Check sheet for the modelled part. Datum: model origin and axes. Units: mm. A direction names the side the tool comes from. Give positions to 0.01 mm unless a question says otherwise; leave off trailing zeros. Order: outer loops, then holes, each group sorted by start corner. A loop starts at its lowest first (then second) coordinate and runs counter-clockwise, first axis right, second up.
from build123d import *

# Parameters (mm, degrees)
SKETCH1_W               = 11.811
SKETCH1_H               = 3.175
SKETCH1_R               = 3.1623
BOSS_EXTRUDE1_DEPTH     = 5.08
BOSS_EXTRUDE2_OUTLINE_W = 16.150142566
BOSS_EXTRUDE2_OUTLINE_H = 6.574737844
BOSS_EXTRUDE2_DEPTH     = 12.7
BOSS_EXTRUDE3_START     = -5.08
BOSS_EXTRUDE3_DEPTH     = 5.08
BOSS_EXTRUDE5_DEPTH     = 2.032
BOSS_EXTRUDE6_START     = -1.27
SKETCH1_6_R             = 5.53085
SKETCH1_6_R_2           = 3.1623
BOSS_EXTRUDE6_DEPTH     = 1.27


# Read off the part's stored shape, not the designer's step: Boss-Extrude2
with BuildPart() as part:
    # Sketch1 → Boss-Extrude1 (new body)
    with BuildSketch(Plane(origin=(0, 0, 0), x_dir=(1, 0, 0), z_dir=(0, 1, 0))):
        with BuildLine():
            ThreePointArc((13.753578899, 4.597841674), (0, 5.078127233), (-13.753578899, 4.597841674))
            Line((-13.753578899, 4.597841674), (-13.39934665, -0.467915496))
            Line((-13.39934665, -0.467915496), (-13.39934665, -22.557024998))
            Line((-13.39934665, -22.557024998), (13.39934665, -22.557024998))
            Line((13.39934665, -22.557024998), (13.39934665, -0.467915496))
            Line((13.39934665, -0.467915496), (13.753578899, 4.597841674))
        make_face()
        with Locations((0, -3.5433)):
            Rectangle(SKETCH1_W, SKETCH1_H, mode=Mode.SUBTRACT)
        with Locations(Location((0, -13.62075, 0), (0, 0, 270))):
            Circle(SKETCH1_R, mode=Mode.SUBTRACT)
    extrude(amount=BOSS_EXTRUDE1_DEPTH)

    # Boss-Extrude2 outline → Boss-Extrude2 (add)
    with BuildSketch(Plane(origin=(0, 0, 0), x_dir=(1, 0, 0), z_dir=(0, 1, 0))):
        with Locations((0, -3.6068)):
            Rectangle(BOSS_EXTRUDE2_OUTLINE_W, BOSS_EXTRUDE2_OUTLINE_H)
        Polygon((-2.8321, -3.6068), (-2.8321, -5.1308), (-5.9055, -5.1308), (-5.9055, -1.9558), (5.9055, -1.9558), (5.9055, -5.1308), (2.8321, -5.1308), (2.8321, -3.6068), align=None, mode=Mode.SUBTRACT)
    extrude(amount=BOSS_EXTRUDE2_DEPTH)

    # Sketch1_4 → Boss-Extrude3 (add)
    with BuildSketch(Plane(origin=(0, 0, 0), x_dir=(1, 0, 0), z_dir=(0, 1, 0)).offset(BOSS_EXTRUDE3_START)):
        with BuildLine():
            ThreePointArc((-13.753578899, 4.597841674), (0, 5.078127233), (13.753578899, 4.597841674))
            Line((13.753578899, 4.597841674), (13.39934665, -0.467915496))
            ThreePointArc((13.39934665, -0.467915496), (6.703757073, -0.117014515), (0, 0))
            ThreePointArc((0, 0), (-6.703757073, -0.117014515), (-13.39934665, -0.467915496))
            Line((-13.39934665, -0.467915496), (-13.753578899, 4.597841674))
        make_face()
    extrude(amount=BOSS_EXTRUDE3_DEPTH)

    # Sketch2 → Boss-Extrude5 (add)
    with BuildSketch(Plane.XZ.offset(5.08)):
        Polygon((-13.753578899, -4.597841674), (-13.39934665, 0.467915496), (-13.300671129, 1.879041191), (13.300671129, 1.879041191), (13.39934665, 0.467915496), (13.753578899, -4.597841674), align=None)
    extrude(amount=-BOSS_EXTRUDE5_DEPTH)

    # Sketch1_6 → Boss-Extrude6 (add)
    with BuildSketch(Plane(origin=(0, 0, 0), x_dir=(1, 0, 0), z_dir=(0, 1, 0)).offset(BOSS_EXTRUDE6_START)):
        with Locations(Location((0, -13.62075, 0), (0, 0, 270))):
            Circle(SKETCH1_6_R)
        with Locations(Location((0, -13.62075, 0), (0, 0, 270))):
            Circle(SKETCH1_6_R_2, mode=Mode.SUBTRACT)
    extrude(amount=BOSS_EXTRUDE6_DEPTH)


solid = part.part
1) Material ranges on L1, parallel to X at y = 3, z = 3.75; L2, parallel to Y at x = 10, z = 1.75; L3, parallel to X at y = 2.5, z = 3.5, recorded low to high.
Recorded:
L1: x = -13.4 to -5.91, -2.83 to 2.83, 5.91 to 13.4
L2: y = -5.08 to -3.05, 0 to 5.08
L3: x = -13.4 to -5.91, 5.91 to 13.4
2) Section check C-C, the plane x = -4.5. Record the cut outline in (y, z).
Recorded:
outline: (-5.08, -5.03) - (5.08, -5.03) - (5.08, 0.32) - (12.7, 0.32) - (12.7, 1.96) - (0, 1.96) - (0, 0.05) - (-3.05, 0.05) - (-3.05, 1.88) - (-5.08, 1.88) - close; (-1.27, 10.41) - (0, 10.41) - (0, 5.13) - (12.7, 5.13) - (12.7, 6.89) - (5.08, 6.89) - (5.08, 22.56) - (0, 22.56) - (0, 16.84) - (-1.27, 16.84) - close
3) Set-up check for faces 1 (the face through (-13.399, 3, 11)), 2 (the face through (8.075, 9, 4)), 3 (the face through (-2.4, -1.27, 16)), 4 (the face through (-5.906, 6, 4)): record each of +Z, -Z, +X, -X, +Y, -Y from which the full face is reachable in a straight line by a thin tool's end or side.
Recorded:
face 1: +Z, -X, +Y, -Y
face 2: +Z, -Z, +X, +Y
face 3: +Z, +X, -X, -Y
face 4: +Y, -Y
4) Draft check along Z on faces 5 (the face through (0, 6, 3.607)), 6 (the face through (-0.19, -0.07, -5.08)), 7 (the face through (-8.075, 9, 4)). Enter one of: +Z half, -Z half, draft (parallel to the pull), parting line (faces both ways), or undercut.
Recorded:
face 5: undercut
face 6: -Z half
face 7: draft
5) Depth check by flat-ended pin: pin 1 Ø1.2 at (y, z) = (5.5, 4.5) entering from -X; pin 2 Ø5 at (x, z) = (1.5, 15.5) entering from +Y; pin 3 Ø4 at (y, z) = (0.5, 15) entering from +X. Enter the tip coordinate at first touch or a pass-through.
Recorded:
pin 1: stops at x = -13.4
pin 2: stops at y = 5.08
pin 3: stops at x = 13.4
6) Section check B-B, the plane y = 8.5. Record the cut outline in (x, z).
Recorded:
outline: (-8.08, 0.32) - (8.08, 0.32) - (8.08, 6.89) - (-8.08, 6.89) - close; hole (-5.91, 1.96) - (5.91, 1.96) - (5.91, 5.13) - (2.83, 5.13) - (2.83, 3.61) - (-2.83, 3.61) - (-2.83, 5.13) - (-5.91, 5.13) - close
7) Section check D-D, the plane z = 12. Record the cut outline in (x, y), then the cut area to 3 significant figures.
Recorded:
outline: (-13.4, 0) - (-5.29, 0) - (-5.29, -1.27) - (-2.72, -1.27) - (-2.72, 5.08) - (-13.4, 5.08) - close; (2.72, -1.27) - (5.29, -1.27) - (5.29, 0) - (13.4, 0) - (13.4, 5.08) - (2.72, 5.08) - close
area: 115 mm2
8) Section check A-A, the plane y = 2.5. Record the cut outline in (x, z).
Recorded:
outline: (-13.75, -4.6) arc R197.17 ccw to (13.75, -4.6) - (13.4, 0.47) - (13.4, 22.56) - (-13.4, 22.56) - (-13.4, 0.47) - close; hole (-5.91, 1.96) - (5.91, 1.96) - (5.91, 5.13) - (2.83, 5.13) - (2.83, 3.61) - (-2.83, 3.61) - (-2.83, 5.13) - (-5.91, 5.13) - close; hole circle Ø6.32 at (0, 13.62)
